Geometry: final body of the model. Coordinates: model frame, mm. Face numbers are marked on the shaded views. A direction names the side the tool comes from. Give positions to 0.01 mm unless a question says otherwise; leave off trailing zeros. Order: outer loops, then holes, each group sorted by start corner. A loop starts at its lowest first (then second) coordinate and runs counter-clockwise, first axis right, second up. Notation, with made-up numbers: (-1.75, 49) -> (26.25, 49) arc R17 ccw to (26.25, 71) -> close; hole circle Ø9 at (36.25, 5.5). An arc over 180 degrees is marked (long way). Answer in a Markdown table with one row per item. Add a question column.
Q1. Cut plane A-A on x = 0. Return the cut outline in (y, z), and give its area (3 significant figures).
Q2. Cut plane B-B on y = -21.5. Return the cut outline in (x, z), and give its area (3 significant figures).
Q3. Cut plane C-C on y = 8.5. Return the cut outline in (x, z), and give its area (3 significant figures).
Q4. Pull-direction query (Y, two-part tool) for the marked faces 5, 6 and 7; classes: +Y half, -Y half, draft (parallel to the pull), parting line (faces both ways), or undercut.
Q5. Set-up query: the marked faces 1, 2, 3 and 4. Return all of +Z, -Z, +X, -X, +Y, -Y with unobstructed straight access to the full face (end or side cutting, diameter ignored); none if empty.
Q6. Contact query for flat-ended pins moving along their axis: P1, Ø5, axis at x = -18, y = -5, coming from the -Z side; P2, Ø1.5, axis at x = 12.5, y = -7.5, coming from the -Z side; P3, Ø5, axis at y = -2.5, z = -7.5, coming from the -X side. Output: stop coordinate, or through.
Q7. Line query: line 1 along Y through (x, z) = (-16.5, -34); line 2 along X through (y, z) = (-10.5, -15.5); line 3 along X through (y, z) = (-28.5, -9). Output: solid intervals per line, ascending. Write a range as from..to.
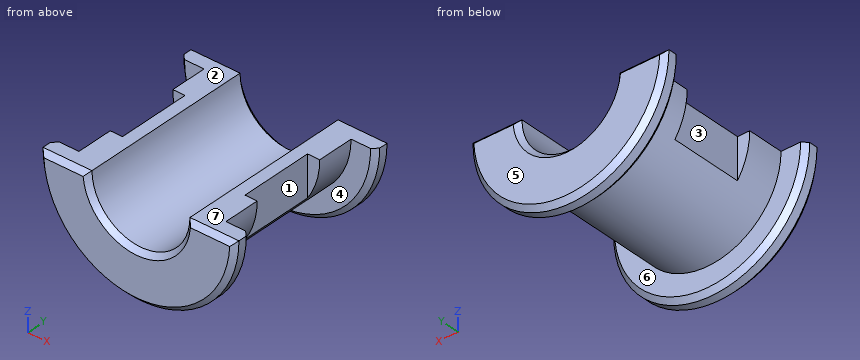
from build123d import *

# Parameters (mm, degrees)
REVOLVE_1_ANGLE     = 180
CUT_EXTRUDE_START   = -30
CUT_EXTRUDE_1_DEPTH = 30
CUT_EXTRUDE_2_DEPTH = 30
HOLE_WIZARD_M39_1_D = 40
CHAMFER_1_SIZE      = 2


with BuildPart() as part:
    # 草图1 → 旋转1 (revolve)
    with BuildSketch(Plane.XY):
        Polygon((0, 37.5), (0, -37.5), (40, -37.5), (40, -30), (30, -30), (30, 29.999999991), (40, 29.999999991), (40, 37.5), align=None)
    revolve(axis=Axis((0, 37.5, 0), (0, 1, 0)), revolution_arc=REVOLVE_1_ANGLE)

    # 草图2 → 切除-拉伸1 (cut)
    with BuildSketch(Plane.XZ.offset(15).offset(CUT_EXTRUDE_START)):
        with BuildLine():
            Line((25, 0), (25, -16.583123956))
            ThreePointArc((25, -16.583123956), (28.722813235, -8.66025404), (30.000000003, 0))
            Line((30.000000003, 0), (25, 0))
        make_face()
    extrude(amount=CUT_EXTRUDE_1_DEPTH, mode=Mode.SUBTRACT)

    # 草图3 → 切除-拉伸2 (cut)
    with BuildSketch(Plane.XZ.offset(15).offset(CUT_EXTRUDE_START)):
        with BuildLine():
            Line((-24.999999999, -16.583123954), (-24.999999999, 0))
            Line((-24.999999999, 0), (-30, 0))
            ThreePointArc((-30, 0), (-28.722813232, -8.660254039), (-24.999999999, -16.583123954))
        make_face()
    extrude(amount=CUT_EXTRUDE_2_DEPTH, mode=Mode.SUBTRACT)

    # M39 螺旋的螺纹孔钻头1 (through all)
    with Locations(Plane(origin=(0, 37.5, 0), x_dir=(1, 0, 0), z_dir=(0, 1, 0))):
        with Locations((0, 0)):
            Hole(HOLE_WIZARD_M39_1_D / 2)

    # 倒角1
    chamfer_1_edges = [part.edges().sort_by_distance(p)[0] for p in [
        (30, -37.5, 0),
        (0, 37.5, -40),
        (0, 29.999999991, -40),
        (0, -30, -40),
        (0, -37.5, -40),
        (-30, 37.5, 0),
        (-30, -37.5, 0),
        (30, 37.5, 0),
        (0, 37.5, -20),
        (0, -37.5, -20),
    ]]
    chamfer(chamfer_1_edges, length=CHAMFER_1_SIZE)


solid = part.part
Completed:
| question | item | result |
|---|---|---|
| 1 | outline | (-37.5, -38) -> (-35.5, -40) -> (-32, -40) -> (-30, -38) -> (-30, -30) -> (30, -30) -> (30, -38) -> (32, -40) -> (35.5, -40) -> (37.5, -38) -> (37.5, -22) -> (35.5, -20) -> (-35.5, -20) -> (-37.5, -22) -> close |
| 1 | area | 888 mm² |
| 2 | outline | (-30, 0) arc R30 ccw to (30, 0) -> (20, 0) arc R20 cw to (-20, 0) -> close |
| 2 | area | 785 mm² |
| 3 | outline | (-25, -16.58) arc R30 ccw to (25, -16.58) -> (25, 0) -> (20, 0) arc R20 cw to (-20, 0) -> (-25, 0) -> close |
| 3 | area | 673 mm² |
| 4 | face 5 | +Y half |
| 4 | face 6 | undercut |
| 4 | face 7 | draft |
| 5 | face 1 | +Z, -Z, +X |
| 5 | face 2 | +Z, +X, -X, +Y, -Y |
| 5 | face 3 | +Z, -Z, -X |
| 5 | face 4 | -Z |
| 6 | P1 | stops at z = -25.69 |
| 6 | P2 | stops at z = -27.6 |
| 6 | P3 | stops at x = -25 |
| 7 | line 1 | y = -37.5..-30, 30..37.5 |
| 7 | line 2 | x = -25..-12.64, 12.64..25 |
| 7 | line 3 | x = -28.62..-17.86, 17.86..28.62 |
